Work out the finished part from the listing and answer in its coordinate system (mm). A direction names the side the tool comes from. Give positions to 0.01 mm unless a question says otherwise; leave off trailing zeros. Order: outer loops, then holes, each group sorted by start corner. A loop starts at its lowest first (then second) coordinate and runs counter-clockwise, first axis right, second up. Notation, with made-up numbers: (36.5, 30) - (40.5, 30) arc R27 cw to (40.5, 53) - close; hole circle Ø11 at (86, 48.25). An arc over 180 degrees is marked (long way). Put each result on its own line as item: value.
```python
from build123d import *

# Parameters (mm, degrees)
ENL_V_MAT_EXTRU_2_REACH = 117.06


with BuildPart() as part:
    # Esquisse1 → Révolution1 (revolve)
    with BuildSketch(Plane.XY, mode=Mode.PRIVATE) as r_volution1_sk:
        Polygon((-76, 0), (-18.5, 0), (-18.5, 14.461538462), (-66, 14.461538462), (-66, 47.461538462), (-76, 47.461538462), (-76, 28.461538462), (-79.5, 28.461538462), (-79.5, 23.461538462), (-76, 23.461538462), align=None)
    revolve(r_volution1_sk.sketch.rotate(Axis((0, 101.923076923, 0), (0, -1, 0)), 270), axis=Axis((0, 101.923076923, 0), (0, -1, 0)))

    # Esquisse2 → Enlèv. mat.-Extru.2 (cut, up to next)
    with BuildSketch(Plane(origin=(0, 24.461538462, 0), x_dir=(1, 0, 0), z_dir=(0, 1, 0)), mode=Mode.PRIVATE) as enl_v_mat_extru_2_sk1:
        with BuildLine():
            Line((-35, 26), (-25, 26))
            ThreePointArc((-25, 26), (-22, 23), (-25, 20))
            Line((-25, 20), (-35, 20))
            ThreePointArc((-35, 20), (-38, 23), (-35, 26))
        make_face()
    enl_v_mat_extru_2_tool1 = extrude(enl_v_mat_extru_2_sk1.sketch, amount=-ENL_V_MAT_EXTRU_2_REACH, mode=Mode.PRIVATE) & part.part
    add(enl_v_mat_extru_2_tool1.solids().sort_by_distance((-30, 24.461538, -23))[0], mode=Mode.SUBTRACT)


solid = part.part
```
(1) Determine the mould class of faces 1 (the face through (-30, 7, -26)), 2 (the face through (46.245, 11.567, -60.311)), 3 (the face through (64.43, 31.19, -14.31)), 4 (the face through (64.4, 28.462, -40.9)) for opening direction Z: pulls with the +Z half, pulls with the -Z half, needs draft (parallel to the pull), parting line crosses it, or undercut.
Geometry check:
face 1: undercut
face 2: parting line crosses it
face 3: undercut
face 4: needs draft
(2) A tool of negligible diameter and unlimited length cuts with its end or side. For faces 5 (the face through (-62.3, 47.462, 22.9)), 6 (the face through (46.245, 37.829, -60.311)), 7 (the face through (40.9, 23.462, 64.4)), 8 (the face through (-30, 7, -20)), from which of +Z, -Z, +X, -X, +Y, -Y can it reach the whole face along a straight path? Write none if from no direction.
Geometry check:
face 5: +Z, -Z, +X, -X, +Y
face 6: +Y
face 7: -Y
face 8: +Y, -Y
(3) Section A-A, the plane z = -2.5 is taken. Write down the section's boundary in (x, y).
Geometry check:
outline: (-79.46, 23.46) - (-75.96, 23.46) - (-75.96, 0) - (-18.33, 0) - (-18.33, 14.46) - (-65.95, 14.46) - (-65.95, 47.46) - (-75.96, 47.46) - (-75.96, 28.46) - (-79.46, 28.46) - close; (18.33, 0) - (75.96, 0) - (75.96, 23.46) - (79.46, 23.46) - (79.46, 28.46) - (75.96, 28.46) - (75.96, 47.46) - (65.95, 47.46) - (65.95, 14.46) - (18.33, 14.46) - close
(4) Given pin 1 (3 mm diameter, centred on x = 47.5, y = 31.5, fed in from +Z); pin 2 (1.5 mm diameter, centred on y = 16.5, z = -38.5, fed in from +X); pin 3 (3 mm diameter, centred on x = -62.5, y = 13, fed in from -Z), each flat-ended and moving along its own axis, determine where each tip first touches the part or whether it passes through.
Geometry check:
pin 1: stops at z = 60.5
pin 2: stops at x = 65.96
pin 3: stops at z = -45.33
(5) Section C-C, the plane x = 4 is taken. Write down the section's boundary in (y, z).
Geometry check:
outline: (0, -75.89) - (23.46, -75.89) - (23.46, -79.4) - (28.46, -79.4) - (28.46, -75.89) - (47.46, -75.89) - (47.46, -65.88) - (14.46, -65.88) - (14.46, -18.06) - (0, -18.06) - close; (0, 18.06) - (14.46, 18.06) - (14.46, 65.88) - (47.46, 65.88) - (47.46, 75.89) - (28.46, 75.89) - (28.46, 79.4) - (23.46, 79.4) - (23.46, 75.89) - (0, 75.89) - close
(6) Straight lines are drawn through the part: line 1 (X direction, y = 32, z = 0); line 2 (Y direction, x = 57.5, z = 16); line 3 (Z direction, x = 53.5, y = 25.5). For each, find the intervals that lie inside material, in ascending order.
Geometry check:
line 1: x = -76 to -66, 66 to 76
line 2: y = 0 to 14.46
line 3: z = -58.8 to -38.65, 38.65 to 58.8
(7) Section D-D, the plane y = 11 is taken. Write down the section's boundary in (x, z), then the cut area to 3 significant figures.
Geometry check:
outline: circle Ø152 at (0, 0); hole (-35, -26) - (-25, -26) arc R3 ccw to (-25, -20) - (-35, -20) arc R3 ccw to start; hole circle Ø37 at (0, 0)
area: 17,000 mm²
(8) Section B-B, the plane y = 37 is taken. Write down the section's boundary in (x, z).
Geometry check:
outline: circle Ø152 at (0, 0); hole circle Ø132 at (0, 0)
